Verification items for the finished model (mm, model axes). A direction names the side the tool comes from. Coordinates: 2 decimals unless noted, no trailing zeros. Loops run counter-clockwise (first coordinate to the right, second up) from the corner with the lowest first, then second, coordinate; pieces in that order, holes last. Notation, with made-up numbers: (61.5, -7.75) -> (68.5, -7.75) arc R16 cw to (68.5, 13.25) -> close; hole circle Ø4 at (58.5, 61). An arc over 180 degrees is marked (long way). Write item = value, one per line.
```python
from build123d import *

# Parameters (mm, degrees)
SKETCH1_R           = 60
BOSS_EXTRUDE1_DEPTH = 4
SKETCH2_R           = 10
CUT_EXTRUDE1_DEPTH  = 85.947042326
SKETCH3_R           = 8.446784488
CUT_EXTRUDE2_DEPTH  = 2.755913
CIRPATTERN1_START   = 1.244087156
CIRPATTERN1_DEPTH   = 2.755912844


# Read off the part's stored shape, not the designer's step: CirPattern1
with BuildPart() as part:
    # Sketch1 → Boss-Extrude1 (new body)
    with BuildSketch(Plane(origin=(0, 0, 0), x_dir=(1, 0, 0), z_dir=(0, 1, 0))):
        with Locations(Location((0, 0, 0), (0, 0, 270))):
            Circle(SKETCH1_R)
    extrude(amount=BOSS_EXTRUDE1_DEPTH)

    # Sketch2 → Cut-Extrude1 (cut, through all)
    with BuildSketch(Plane(origin=(0, 0, 0), x_dir=(1, 0, 0), z_dir=(0, 1, 0))):
        with Locations(Location((0, 0, 0), (0, 0, 270))):
            Circle(SKETCH2_R)
    extrude(amount=CUT_EXTRUDE1_DEPTH, mode=Mode.SUBTRACT)

    # Sketch3 → Cut-Extrude2 (cut)
    with BuildSketch(Plane(origin=(0, 4, 0), x_dir=(1, 0, 0), z_dir=(0, 1, 0))):
        with Locations((-18.16438515, 0)):
            Circle(SKETCH3_R)
    extrude(amount=-CUT_EXTRUDE2_DEPTH, mode=Mode.SUBTRACT)

    # CirPattern1 outline → CirPattern1 (cut)
    with BuildSketch(Plane(origin=(0, 0, 0), x_dir=(1, 0, 0), z_dir=(0, 1, 0)).offset(CIRPATTERN1_START)):
        with BuildLine():
            ThreePointArc((1.601825051, -9.870874151), (0, -10), (-1.601825051, -9.870874151))
            ThreePointArc((-1.601825051, -9.870874151), (-3.151365064, -10.327481015), (-4.585643686, -11.070723178))
            ThreePointArc((-4.585643686, -11.070723178), (-5.074280252, -9.530983465), (-5.847100693, -8.112423404))
            ThreePointArc((-5.847100693, -8.112423404), (-7.071067812, -7.071067812), (-8.112423404, -5.847100693))
            ThreePointArc((-8.112423404, -5.847100693), (-9.530983465, -5.074280252), (-11.070723178, -4.585643686))
            ThreePointArc((-11.070723178, -4.585643686), (-14.93194067, -7.803811305), (-19.937821889, -8.25851623))
            ThreePointArc((-19.937821889, -8.25851623), (-18.816938507, -18.816938507), (-8.25851623, -19.937821889))
            ThreePointArc((-8.25851623, -19.937821889), (0, -26.611169639), (8.25851623, -19.937821889))
            ThreePointArc((8.25851623, -19.937821889), (18.816938507, -18.816938507), (19.937821889, -8.25851623))
            ThreePointArc((19.937821889, -8.25851623), (26.611169639, 0), (19.937821889, 8.25851623))
            ThreePointArc((19.937821889, 8.25851623), (18.816938507, 18.816938507), (8.25851623, 19.937821889))
            ThreePointArc((8.25851623, 19.937821889), (0, 26.611169639), (-8.25851623, 19.937821889))
            ThreePointArc((-8.25851623, 19.937821889), (-18.816938507, 18.816938507), (-19.937821889, 8.25851623))
            ThreePointArc((-19.937821889, 8.25851623), (-14.93194067, 7.803811305), (-11.070723178, 4.585643686))
            ThreePointArc((-11.070723178, 4.585643686), (-9.530983465, 5.074280252), (-8.112423404, 5.847100693))
            ThreePointArc((-8.112423404, 5.847100693), (-7.071067812, 7.071067812), (-5.847100693, 8.112423404))
            ThreePointArc((-5.847100693, 8.112423404), (-5.074280252, 9.530983465), (-4.585643686, 11.070723178))
            ThreePointArc((-4.585643686, 11.070723178), (-3.151365064, 10.327481015), (-1.601825051, 9.870874151))
            ThreePointArc((-1.601825051, 9.870874151), (0, 10), (1.601825051, 9.870874151))
            ThreePointArc((1.601825051, 9.870874151), (3.151365064, 10.327481015), (4.585643686, 11.070723178))
            ThreePointArc((4.585643686, 11.070723178), (5.074280252, 9.530983465), (5.847100693, 8.112423404))
            ThreePointArc((5.847100693, 8.112423404), (7.071067812, 7.071067812), (8.112423404, 5.847100693))
            ThreePointArc((8.112423404, 5.847100693), (9.530983465, 5.074280252), (11.070723178, 4.585643686))
            ThreePointArc((11.070723178, 4.585643686), (10.327481015, 3.151365064), (9.870874151, 1.601825051))
            ThreePointArc((9.870874151, 1.601825051), (10, 0), (9.870874151, -1.601825051))
            ThreePointArc((9.870874151, -1.601825051), (10.327481015, -3.151365064), (11.070723178, -4.585643686))
            ThreePointArc((11.070723178, -4.585643686), (9.530983465, -5.074280252), (8.112423404, -5.847100693))
            ThreePointArc((8.112423404, -5.847100693), (7.071067812, -7.071067812), (5.847100693, -8.112423404))
            ThreePointArc((5.847100693, -8.112423404), (5.074280252, -9.530983465), (4.585643686, -11.070723178))
            ThreePointArc((4.585643686, -11.070723178), (3.151365064, -10.327481015), (1.601825051, -9.870874151))
        make_face()
    extrude(amount=CIRPATTERN1_DEPTH, mode=Mode.SUBTRACT)


solid = part.part
```
1) Sectioned sample at B-B, the plane z = 0. Record the cut outline in (x, y), plus the area to 3 significant figures.
Ans:
outline = (-60, 0) -> (-10, 0) -> (-10, 1.24) -> (-26.61, 1.24) -> (-26.61, 4) -> (-60, 4) -> close; (10, 0) -> (60, 0) -> (60, 4) -> (26.61, 4) -> (26.61, 1.24) -> (10, 1.24) -> close
area = 308 mm2
2) Material ranges on line 1 (X direction, y = 2.3, z = 0); line 2 (Z direction, x = 9, y = 3.05); line 3 (X direction, y = 1.05, z = 0), recorded low to high.
Ans:
line_1 = -60 to -26.61, 26.61 to 60
line_2 = -59.32 to -20.37, -5.32 to -4.36, 4.36 to 5.32, 20.37 to 59.32
line_3 = -60 to -10, 10 to 60
3) Sectioned sample at A-A, the plane y = 2.8. Count the separate pieces of the cut face and the enclosed holes in it, plus the area to 3 significant figures.
Ans:
separate_pieces = 9
enclosed_holes = 1
area = 9,360 mm2
4) Sectioned sample at C-C, the plane x = 0. Record the cut outline in (y, z).
Ans:
outline = (0, -60) -> (4, -60) -> (4, -26.61) -> (1.24, -26.61) -> (1.24, -10) -> (0, -10) -> close; (0, 10) -> (1.24, 10) -> (1.24, 26.61) -> (4, 26.61) -> (4, 60) -> (0, 60) -> close
5) Sectioned sample at D-D, the plane z = 18.5. Record the cut outline in (x, y).
Ans:
outline = (-57.08, 0) -> (57.08, 0) -> (57.08, 4) -> (19.12, 4) -> (19.12, 1.24) -> (-19.12, 1.24) -> (-19.12, 4) -> (-57.08, 4) -> close
6) Release check for a two-part mould opening along Z. For faces 1 (the face through (18.7, 2.6, 18.93)), 2 (the face through (4, 4, -10)) record: pulls with the +Z half, pulls with the -Z half, needs draft (parallel to the pull), parting line crosses it, or undercut.
Ans:
face_1 = undercut
face_2 = needs draft
7) Tool access check on faces 3 (the face through (-10, 4, -4)), 4 (the face through (-3.13, 2.6, 10.32)). Record the directions out of +Z, -Z, +X, -X, +Y, -Y that give a thin tool (end or side, any length) a straight path to the whole face; none if there is none.
Ans:
face_3 = +Z, -Z, +X, -X, +Y
face_4 = +Y
